```python
from build123d import *
from OCP.BRepFilletAPI import BRepFilletAPI_MakeChamfer

# Parameters (mm, degrees)
SKETCH_1_R       = 1
SKETCH_1_R_2     = 5
EXTRUDE_1_DEPTH  = 2.5
EXTRUDE_START    = 2.5
SKETCH_1_3_R     = 5
EXTRUDE_2_DEPTH  = 1
EXTRUDE_START_2  = -1
SKETCH_1_4_R     = 5
EXTRUDE_3_DEPTH  = 1
EXTRUDE_START_3  = -2.5
SKETCH_1_5_R     = 5
SKETCH_1_5_R_2   = 3.5
SKETCH_1_5_R_3   = 3
EXTRUDE_4_DEPTH  = 2.5
CHAMFER_1_SIZE   = 2
CHAMFER_1_SIZE_2 = 1
CHAMFER_2_SIZE   = 1


with BuildPart() as part:
    # Эскиз1 → Бобышка-Вытянуть1 (new body)
    # profile 1 of 2: a face of its own
    with BuildSketch(Plane(origin=(0, 0, 0), x_dir=(1, 0, 0), z_dir=(0, 1, 0))):
        with BuildLine():
            ThreePointArc((-29.362068966, 3.481221921), (-32.5, 0), (-29.362068966, -3.481221921))
            Line((-29.362068966, -3.481221921), (-9.951914627, -5.5))
            Line((-9.951914627, -5.5), (-9.951914627, 5.5))
            Line((-9.951914627, 5.5), (-29.362068966, 3.481221921))
        make_face()
        with Locations(Location((-29, 0, 0), (0, 0, 270))):
            Circle(SKETCH_1_R, mode=Mode.SUBTRACT)
        with Locations(Location((-26, 0, 0), (0, 0, 270))):
            Circle(SKETCH_1_R, mode=Mode.SUBTRACT)
        with Locations(Location((-23, 0, 0), (0, 0, 270))):
            Circle(SKETCH_1_R, mode=Mode.SUBTRACT)
        with Locations(Location((-20, 0, 0), (0, 0, 270))):
            Circle(SKETCH_1_R, mode=Mode.SUBTRACT)
        with Locations(Location((-17, 0, 0), (0, 0, 270))):
            Circle(SKETCH_1_R, mode=Mode.SUBTRACT)
        with Locations(Location((-14, 0, 0), (0, 0, 270))):
            Circle(SKETCH_1_R, mode=Mode.SUBTRACT)
    # profile 2 of 2: a face of its own
    with BuildSketch(Plane(origin=(0, 0, 0), x_dir=(1, 0, 0), z_dir=(0, 1, 0))):
        with BuildLine():
            Line((-9.951914627, 5.5), (-9.951914627, -5.5))
            Line((-9.951914627, -5.5), (-0.672413793, -6.465126425))
            ThreePointArc((-0.672413793, -6.465126425), (6.5, 0), (-0.672413793, 6.465126425))
            Line((-0.672413793, 6.465126425), (-9.951914627, 5.5))
        make_face()
        with Locations(Location((0, 0, 0), (0, 0, 270))):
            Circle(SKETCH_1_R_2, mode=Mode.SUBTRACT)
    extrude(amount=EXTRUDE_1_DEPTH)

    # Эскиз1<3> → Бобышка-Вытянуть2 (add)
    with BuildSketch(Plane(origin=(0, 0, 0), x_dir=(1, 0, 0), z_dir=(0, 1, 0)).offset(EXTRUDE_START)):
        with BuildLine():
            Line((-9.951914627, 5.5), (-9.951914627, -5.5))
            Line((-9.951914627, -5.5), (-0.672413793, -6.465126425))
            ThreePointArc((-0.672413793, -6.465126425), (6.5, 0), (-0.672413793, 6.465126425))
            Line((-0.672413793, 6.465126425), (-9.951914627, 5.5))
        make_face()
        with Locations(Location((0, 0, 0), (0, 0, 270))):
            Circle(SKETCH_1_3_R, mode=Mode.SUBTRACT)
    extrude(amount=EXTRUDE_2_DEPTH)

    # Эскиз1<4> → Бобышка-Вытянуть3 (add)
    with BuildSketch(Plane(origin=(0, 0, 0), x_dir=(1, 0, 0), z_dir=(0, 1, 0)).offset(EXTRUDE_START_2)):
        with BuildLine():
            Line((-9.951914627, 5.5), (-9.951914627, -5.5))
            Line((-9.951914627, -5.5), (-0.672413793, -6.465126425))
            ThreePointArc((-0.672413793, -6.465126425), (6.5, 0), (-0.672413793, 6.465126425))
            Line((-0.672413793, 6.465126425), (-9.951914627, 5.5))
        make_face()
        with Locations(Location((0, 0, 0), (0, 0, 270))):
            Circle(SKETCH_1_4_R, mode=Mode.SUBTRACT)
    extrude(amount=EXTRUDE_3_DEPTH)

    # Эскиз1<5> → Бобышка-Вытянуть4 (add)
    # profile 1 of 2: a face of its own
    with BuildSketch(Plane(origin=(0, 0, 0), x_dir=(1, 0, 0), z_dir=(0, 1, 0)).offset(EXTRUDE_START_3)):
        with Locations(Location((0, 0, 0), (0, 0, 270))):
            Circle(SKETCH_1_5_R)
        Circle(SKETCH_1_5_R_2, mode=Mode.SUBTRACT)
    # profile 2 of 2: a face of its own
    with BuildSketch(Plane(origin=(0, 0, 0), x_dir=(1, 0, 0), z_dir=(0, 1, 0)).offset(EXTRUDE_START_3)):
        Circle(SKETCH_1_5_R_2)
        with Locations(Location((0, 0, 0), (0, 0, 270))):
            Circle(SKETCH_1_5_R_3, mode=Mode.SUBTRACT)
    extrude(amount=EXTRUDE_4_DEPTH)

    # Фаска1
    chamfer_1_edges_1 = [part.edges().sort_by_distance(p)[0] for p in [
        (-9.951914627, 3.5, 0),
    ]]
    chamfer_1_side_1 = [part.faces().sort_by_distance(p)[0] for p in [
        (-9.931914627, 3.5, 0),
    ]]
    chamfer_1_edges_2 = [part.edges().sort_by_distance(p)[0] for p in [
        (-9.951914627, -1, 0),
    ]]
    chamfer_1_side_2 = [part.faces().sort_by_distance(p)[0] for p in [
        (-9.951914627, -0.98, 0),
    ]]
    chamfer_1 = BRepFilletAPI_MakeChamfer(part.part.solid().wrapped)
    for e in chamfer_1_edges_1:
        chamfer_1.Add(CHAMFER_1_SIZE - 0.0001, CHAMFER_1_SIZE_2 - 0.0001, e.wrapped, chamfer_1_side_1[0].wrapped)
    for e in chamfer_1_edges_2:
        chamfer_1.Add(CHAMFER_1_SIZE_2 - 0.0001, CHAMFER_1_SIZE - 0.0001, e.wrapped, chamfer_1_side_2[0].wrapped)
    add(Compound.cast(chamfer_1.Shape()), mode=Mode.REPLACE)  # a hair under: the kernel refuses the full size

    # Фаска2
    chamfer_2_edges = [part.edges().sort_by_distance(p)[0] for p in [
        (0, -2.5, -5),
    ]]
    chamfer(chamfer_2_edges, length=CHAMFER_2_SIZE)


solid = part.part
```
Check sheet for the modelled part. Datum: model origin and axes. Units: mm. A direction names the side the tool comes from. Round coordinates to 2 decimals unless told otherwise and drop trailing zeros. Loops run counter-clockwise (first coordinate to the right, second up) from the corner with the lowest first, then second, coordinate; pieces in that order, holes last. Notation, with made-up numbers: (39.25, -4.5) - (83.25, -4.5) arc R18 cw to (83.25, 16.5) - close; hole circle Ø8 at (-23.75, -33). An arc over 180 degrees is marked (long way). Write item = value, one per line. Start each with the question number.
Q1. Section check B-B (x = 0). Record the boundary of the cut face in (y, z).
Q2. Depth check by flat-ended pin: P1, Ø3, axis at x = -29, z = 0, coming from the +Y side; P2, Ø1, axis at x = -18, z = 0.5, coming from the -Y side; P3, Ø1, axis at x = -14.5, y = 1, coming from the +Z side. Enter the tip coordinate at first touch or a pass-through.
Q3. Thickness scan on L1, parallel to Y at x = -0.5, z = -3; L2, parallel to Y at x = -28, z = -3.25; L3, parallel to Z at x = -4, y = -1.25. Record the ranges inside material, lowest first.
Q4. Access from +Z, -Z, +X, -X, +Y, -Y to the whole of each face (thin tool, end or side, straight path). Record for faces 1 (the face through (-21, 1, 0)), 2 (the face through (-21.4, 0, -0.1)), 3 (the face through (-0.1, 0, 3.3)), 4 (the face through (-21.4, 2.5, -0.1)), 5 (the face through (-6, -1, 0)).
Q5. Section check C-C (z = 0). Count the separate pieces of the cut face and the enclosed holes in it, plus the area to 3 significant figures.
Q6. Section check D-D (y = -0.5). Record the boundary of the cut face in (x, z), plus the area to 3 significant figures.
Q7. Section check A-A (y = 1.75). Record the boundary of the cut face in (x, z), plus the area to 3 significant figures.
Q8. Release check for a two-part mould opening along Z. For faces 6 (the face through (-8.97, 2.99, -0.08)), 7 (the face through (-32.5, 1.2, -0.1)), 8 (the face through (-4.88, 1.73, -1.08)) record: pulls with the +Z half, pulls with the -Z half, needs draft (parallel to the pull), parting line crosses it, or undercut.
Derived:
q1.outline = (-2.5, -4) - (-1.5, -5) - (-1, -5) - (-1, -6.5) - (3.5, -6.5) - (3.5, -5) - (0, -5) - (0, -3) - (-2.5, -3) - close; (-2.5, 3) - (0, 3) - (0, 5) - (3.5, 5) - (3.5, 6.5) - (-1, 6.5) - (-1, 5) - (-1.5, 5) - (-2.5, 4) - close
q2.P1 = 2.5
q2.P2 = 0
q2.P3 = 5.08
q3.L1 = -2.5 to 0
q3.L2 = 0 to 2.5
q3.L3 = -3 to 3
q4.face_1 = +Y, -Y
q4.face_2 = +Z, -Z, -X, -Y
q4.face_3 = +Y
q4.face_4 = +Z, -Z, -X, +Y
q4.face_5 = -Y
q5.separate_pieces = 8
q5.enclosed_holes = 0
q5.area = 62.4 mm^2
q6.outline = (-8.95, -5.6) - (-0.67, -6.47) arc R6.5 ccw (long way) to (-0.67, 6.47) - (-8.95, 5.6) - close; hole circle Ø6 at (0, 0)
q6.area = 147 mm^2
q7.outline = (-29.36, -3.48) - (-0.67, -6.47) arc R6.5 ccw (long way) to (-0.67, 6.47) - (-29.36, 3.48) arc R3.5 ccw to start; hole circle Ø2 at (-29, 0); hole circle Ø2 at (-26, 0); hole circle Ø2 at (-23, 0); hole circle Ø2 at (-20, 0); hole circle Ø2 at (-17, 0); hole circle Ø2 at (-14, 0); hole circle Ø10 at (0, 0)
q7.area = 280 mm^2
q8.face_6 = needs draft
q8.face_7 = parting line crosses it
q8.face_8 = undercut
